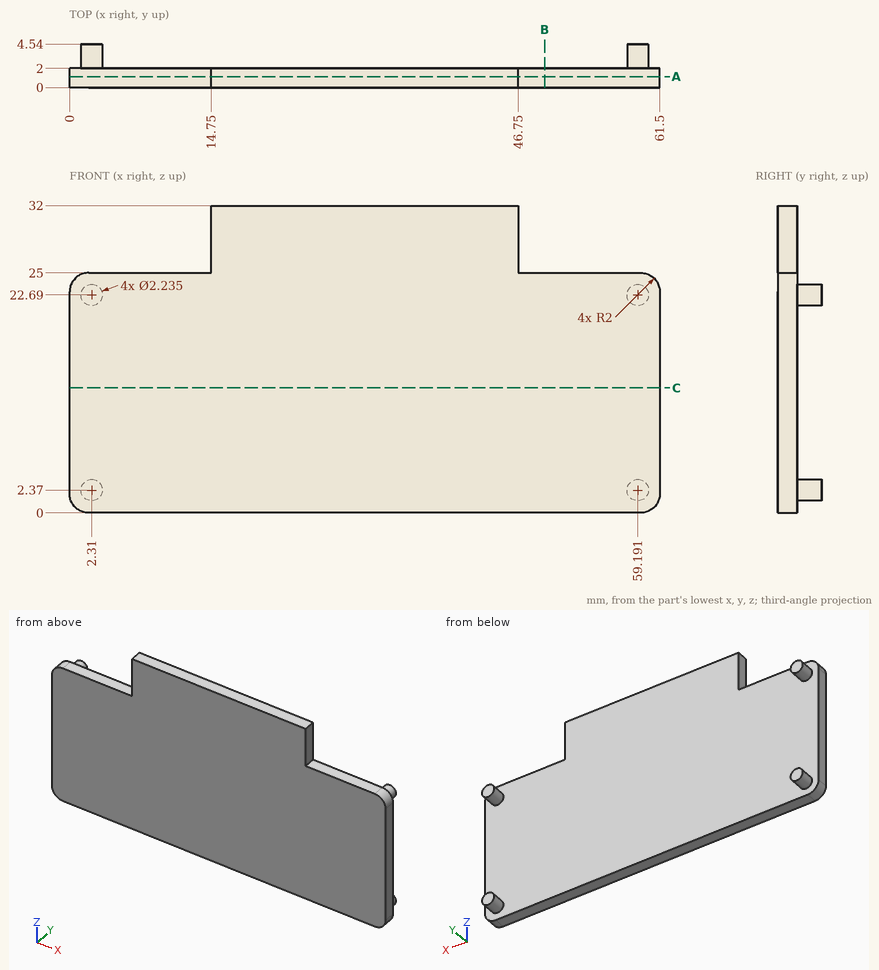
Study the drawing (mm; zero at the part's minimum x, y, z) and answer. Give positions to 0.01 mm unless a question says otherwise; leave off trailing zeros. Write each loop counter-clockwise with the first axis right and the second up, starting at its lowest first coordinate (ties: lowest second). Pieces come first, ordered by that corner, then holes. Notation, with made-up numbers: (51, 19.5) - (101, 19.5) arc R23 cw to (101, 44.5) - close; hole circle Ø10 at (-25, -9.5). An arc over 180 degrees is marked (long way). Write item = value, one per line. Start each with the question number.
Item 1: Find section A-A (y = 1.15). Give the vertices of the cut face in (x, z), then the cut area to 3 significant figures.
Item 2: Find section B-B (x = 49.5). Give the vertices of the cut face in (y, z).
Item 3: Find section C-C (z = 13). Give the vertices of the cut face in (x, y).
Item 4: Each of these flat-tipped pins is pushed along its axis until it touches: P1, Ø1.6, axis at x = 7.5, y = 0.5, coming from the +Z side; P2, Ø3, axis at x = 14, z = 10.5, coming from the -Y side; P3, Ø12, axis at x = 15, z = 5.5, coming from the +Y side; P4, Ø1.6, axis at y = 1, z = 29.5, coming from the +X side. Where does it stop, or does it pass through?
Item 5: Find the intervals of material crossed by probe 1 along X at (y, z) = (1, 26.5); probe 2 along Y at (x, z) = (9, 4.5); probe 3 along Z at (x, y) = (3.5, 0.9), in increasing order. Write a range as [from, to].
Response:
q1.outline = (0, 2) arc R2 ccw to (2, 0) - (59.5, 0) arc R2 ccw to (61.5, 2) - (61.5, 23) arc R2 ccw to (59.5, 25) - (46.75, 25) - (46.75, 32) - (14.75, 32) - (14.75, 25) - (2, 25) arc R2 ccw to (0, 23) - close
q1.area = 1,760 mm²
q2.outline = (0, 0) - (2, 0) - (2, 25) - (0, 25) - close
q3.outline = (0, 0) - (61.5, 0) - (61.5, 2) - (0, 2) - close
q4.P1 = 25
q4.P2 = 0
q4.P3 = 2
q4.P4 = 46.75
q5.probe_1 = [14.75, 46.75]
q5.probe_2 = [0, 2]
q5.probe_3 = [0, 25]
